from build123d import *

# Parameters (mm, degrees)
SKETCH_W     = 32
SKETCH_H     = 47.5
SKETCH_R     = 1.65
PAD_DEPTH    = 3
SKETCH001_W  = 61.411388
SKETCH001_H  = 6.4
POCKET_DEPTH = 1


with BuildPart() as part:
    # Sketch → Pad (new body)
    with BuildSketch(Plane.XY):
        with Locations((0, -10.25)):
            Rectangle(SKETCH_W, SKETCH_H)
        with Locations((-10, -10)):
            Circle(SKETCH_R, mode=Mode.SUBTRACT)
        with Locations((-10, 10)):
            Circle(SKETCH_R, mode=Mode.SUBTRACT)
        with Locations((10, 10)):
            Circle(SKETCH_R, mode=Mode.SUBTRACT)
        with Locations((10, -10)):
            Circle(SKETCH_R, mode=Mode.SUBTRACT)
        with Locations((-11, -17)):
            Circle(SKETCH_R, mode=Mode.SUBTRACT)
        with Locations((11, -17)):
            Circle(SKETCH_R, mode=Mode.SUBTRACT)
        with Locations((-11, -30.4)):
            Circle(SKETCH_R, mode=Mode.SUBTRACT)
        with Locations((11, -30.4)):
            Circle(SKETCH_R, mode=Mode.SUBTRACT)
    extrude(amount=PAD_DEPTH)

    # Sketch001 (on Face14 of Pad) → Pocket (cut)
    with BuildSketch(Plane.XY.offset(3)):
        with Locations((0.476776, -23.7)):
            Rectangle(SKETCH001_W, SKETCH001_H)
    extrude(amount=-POCKET_DEPTH, mode=Mode.SUBTRACT)


solid = part.part
Could you check a few things on this model? Use its own coordinates, in mm. A direction names the side the tool comes from. Round coordinates to 2 decimals unless told otherwise and drop trailing zeros. Order: outer loops, then holes, each group sorted by start corner. A loop starts at its lowest first (then second) coordinate and runs counter-clockwise, first axis right, second up.
(1) Imagine slicing it at A-A (z = 1.1). Count the separate pieces of the cut face and the enclosed holes in it, plus the area to 3 significant figures.
Response values:
separate pieces: 1
enclosed holes: 8
area: 1,450 mm2
(2) Imagine slicing it at D-D (x = -11). Write out the boundary of the cut face in (y, z), plus the area to 3 significant figures.
Response values:
outline: (-34, 0) - (-32.05, 0) - (-32.05, 3) - (-34, 3) - close; (-28.75, 0) - (-18.65, 0) - (-18.65, 3) - (-20.5, 3) - (-20.5, 2) - (-26.9, 2) - (-26.9, 3) - (-28.75, 3) - close; (-15.35, 0) - (-11.31, 0) - (-11.31, 3) - (-15.35, 3) - close; (-8.69, 0) - (8.69, 0) - (8.69, 3) - (-8.69, 3) - close; (11.31, 0) - (13.5, 0) - (13.5, 3) - (11.31, 3) - close
area: 101 mm2
(3) I'm going to push flat-ended pins straight in: pin 1 (6 mm diameter, centred on x = 7, y = -24, fed in from -Z); pin 2 (1.9 mm diameter, centred on x = 0, y = -22.5, fed in from +Z). Where does each tip first touch, or does it pass through?
Response values:
pin 1: stops at z = 0
pin 2: stops at z = 2
(4) If we mould it in two halves opening along X, with no side actions, what happens to faces 1 (the cylindrical face through (-11.4, -32, 1.5)), 2 (the flat face through (-16, -11, 1)), 3 (the cylindrical face through (-9.239, -11.464, 1.479)), 4 (the flat face through (0, -34, 1))? For each: released by +X, released by -X, zero draft, split by the parting line, or undercut.
Response values:
face 1: undercut
face 2: released by -X
face 3: undercut
face 4: zero draft
(5) Imagine slicing it at C-C (x = 0). Write out the boundary of the cut face in (y, z).
Response values:
outline: (-34, 0) - (13.5, 0) - (13.5, 3) - (-20.5, 3) - (-20.5, 2) - (-26.9, 2) - (-26.9, 3) - (-34, 3) - close
(6) Which directions (+Z, -Z, +X, -X, +Y, -Y) give clear straight access to the entire face, cutting with the end or side of a thin tool? Please do faces 5 (the flat face through (0, -30, 3)), 6 (the flat face through (0, -24, 2)).
Response values:
face 5: +Z, +X, -X, +Y, -Y
face 6: +Z, +X, -X
(7) Please list where these lines run through material, in increasing order: line 1 along Y through (x, z) = (10, 1.8); line 2 along X through (y, z) = (-30, 1.55); line 3 along Y through (x, z) = (11, 2.35).
Response values:
line 1: y = -34 to -31.71, -29.09 to -18.31, -15.69 to -11.65, -8.35 to 8.35, 11.65 to 13.5
line 2: x = -16 to -12.6, -9.4 to 9.4, 12.6 to 16
line 3: y = -34 to -32.05, -28.75 to -26.9, -20.5 to -18.65, -15.35 to -11.31, -8.69 to 8.69, 11.31 to 13.5
(8) Imagine slicing it at B-B (y = -17). Write out the boundary of the cut face in (x, z), plus the area to 3 significant figures.
Response values:
outline: (-16, 0) - (-12.65, 0) - (-12.65, 3) - (-16, 3) - close; (-9.35, 0) - (9.35, 0) - (9.35, 3) - (-9.35, 3) - close; (12.65, 0) - (16, 0) - (16, 3) - (12.65, 3) - close
area: 76.2 mm2
